from build123d import *

# Parameters (mm, degrees)
SKETCH1_W           = 13.65
SKETCH1_H           = 1
BOSS_EXTRUDE1_DEPTH = 16.5
SKETCH2_R           = 1.325
BOSS_EXTRUDE2_DEPTH = 11.75


with BuildPart() as part:
    # Sketch1 → Boss-Extrude1 (new body)
    with BuildSketch(Plane(origin=(0, 0, 0), x_dir=(1, 0, 0), z_dir=(0, 1, 0))):
        Rectangle(SKETCH1_W, SKETCH1_H)
    extrude(amount=BOSS_EXTRUDE1_DEPTH)

    # Sketch2 → Boss-Extrude2 (add, symmetric)
    with BuildSketch(Plane(origin=(0, 8.25, 0), x_dir=(1, 0, 0), z_dir=(0, 1, 0))):
        with Locations(Location((-6.825, 0, 0), (0, 0, 270))):
            Circle(SKETCH2_R)
        with Locations(Location((6.825, 0, 0), (0, 0, 270))):
            Circle(SKETCH2_R)
    extrude(amount=BOSS_EXTRUDE2_DEPTH, both=True)


solid = part.part
Geometry check sheet. Reference: the model listing, model coordinates, mm. A direction names the side the tool comes from. Round coordinates to 2 decimals unless told otherwise and drop trailing zeros. Write each loop counter-clockwise with the first axis right and the second up, starting at its lowest first coordinate (ties: lowest second). Pieces come first, ordered by that corner, then holes. Notation, with made-up numbers: (-23, 63) - (-17, 63) arc R15 cw to (-17, 79) - close; hole circle Ø2 at (-39.75, 35). An arc over 180 degrees is marked (long way). One line per item, written item: value.
1. Mould release check, pull along X, two halves, no side actions. Record for faces 4 (the face through (7.942, 8.414, 0.712)), 5 (the face through (7, -3.5, 0)): released by +X, released by -X, zero draft, split by the parting line, or undercut.
The answers:
face 4: undercut
face 5: zero draft
2. Scan lines: L1, parallel to X at y = 3, z = -0.1; L2, parallel to Y at x = -3.5, z = -0.2; L3, parallel to Z at x = -1.25, y = 11. Record each from-to range of solid material in increasing order.
The answers:
L1: x = -8.15 to 8.15
L2: y = 0 to 16.5
L3: z = -0.5 to 0.5
3. Cross-section at C-C on x = 4. Record the boundary of the cut face in (y, z), and give its area (3 significant figures).
The answers:
outline: (0, -0.5) - (16.5, -0.5) - (16.5, 0.5) - (0, 0.5) - close
area: 16.5 mm^2
4. Cross-section at B-B on y = 10. Record the boundary of the cut face in (x, z) (3 decimals), and give its area (3 significant figures).
The answers:
outline: (-5.598, -0.5) - (5.598, -0.5) arc R1.325 ccw (long way) to (5.598, 0.5) - (-5.598, 0.5) arc R1.325 ccw (long way) to start
area: 22.1 mm^2
5. Set-up check for faces 1 (the face through (0, 8, -0.5)), 2 (the face through (0, 8, 0.5)), 3 (the face through (0, 16.5, 0)): record each of +Z, -Z, +X, -X, +Y, -Y from which the full face is reachable in a straight line by a thin tool's end or side.
The answers:
face 1: -Z, +Y, -Y
face 2: +Z, +Y, -Y
face 3: +Z, -Z, +Y
6. Cross-section at A-A on z = 0. Record the boundary of the cut face in (x, y).
The answers:
outline: (-8.15, -3.5) - (-5.5, -3.5) - (-5.5, 0) - (5.5, 0) - (5.5, -3.5) - (8.15, -3.5) - (8.15, 20) - (5.5, 20) - (5.5, 16.5) - (-5.5, 16.5) - (-5.5, 20) - (-8.15, 20) - close
7. Depth check by flat-ended pin: pin 1 Ø0.8 at (x, z) = (-1, 0) entering from -Y; pin 2 Ø1 at (x, y) = (6, 0.5) entering from -Z; pin 3 Ø0.8 at (x, z) = (-1, 0) entering from +Y. Enter the tip coordinate at first touch or a pass-through.
The answers:
pin 1: stops at y = 0
pin 2: stops at z = -1.28
pin 3: stops at y = 16.5
